Check sheet for the drawn part. Datum: minimum x, y, z corner. Units: mm. A direction names the side the tool comes from. Coordinates: 2 decimals unless noted, no trailing zeros. Write each loop counter-clockwise with the first axis right and the second up, starting at its lowest first coordinate (ties: lowest second). Pieces come first, ordered by that corner, then holes. Notation, with made-up numbers: (-34.5, 67.5) - (14.5, 67.5) arc R14 cw to (14.5, 76.5) - close; hole circle Ø9 at (-28, -29). An arc over 180 degrees is marked (long way). Answer as CSV lines item,"result". Start each with the question number.
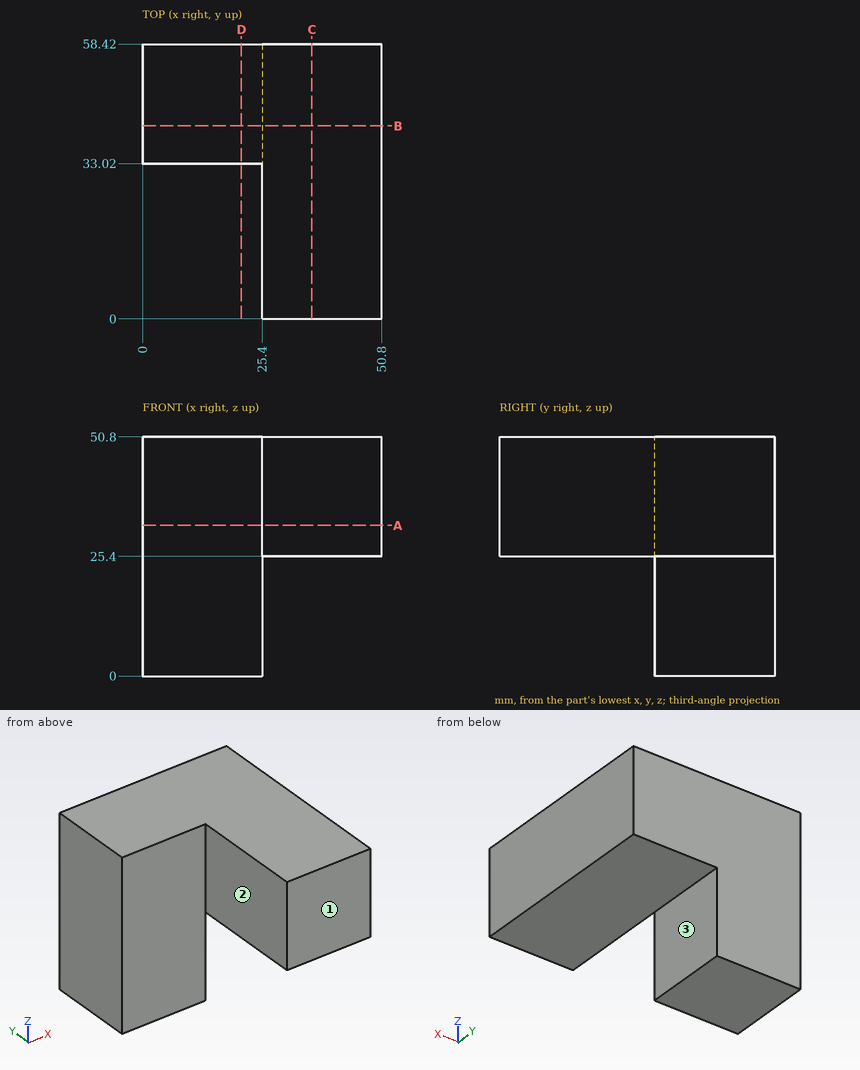
(1) Material ranges on probe 1 along X at (y, z) = (11.5, 26); probe 2 along X at (y, z) = (49.5, 4), recorded low to high. Write a range as from..to.
(2) Go/stop test with flat-tipped pins: P1, Ø12.5, axis at x = 10, z = 13, coming from the -Y side; P2, Ø3, axis at x = 29.5, z = 24.5, coming from the -Y side; P3, Ø2, axis at x = 36, y = 31.5, coming from the -Z side; P4, Ø7.5, axis at y = 12.5, z = 39.5, coming from the -X side. Record where each tip stops, or that it passes through.
(3) Cross-section at D-D on x = 21. Record the boundary of the cut face in (y, z).
(4) Cross-section at B-B on y = 41. Record the boundary of the cut face in (x, z), plus the area to 3 significant figures.
(5) Tool access check on the marked faces 1, 2 and 3. Record the directions out of +Z, -Z, +X, -X, +Y, -Y that give a thin tool (end or side, any length) a straight path to the whole face; none if there is none.
(6) Cross-section at C-C on x = 36. Record the boundary of the cut face in (y, z).
(7) Cross-section at A-A on z = 32. Record the boundary of the cut face in (x, y), plus the area to 3 significant figures.
Checked values:
1,probe 1,"25.4..50.8"
1,probe 2,"0..25.4"
2,P1,"y = 33.02"
2,P2,"y = 0"
2,P3,"z = 25.4"
2,P4,"x = 25.4"
3,outline,"(33.02, 0) - (58.42, 0) - (58.42, 50.8) - (33.02, 50.8) - close"
4,outline,"(0, 0) - (25.4, 0) - (25.4, 25.4) - (50.8, 25.4) - (50.8, 50.8) - (0, 50.8) - close"
4,area,"1,940 mm^2"
5,face 1,"+Z, -Z, +X, -X, -Y"
5,face 2,"+Z, -Z, -X, -Y"
5,face 3,"-Z, +X, +Y, -Y"
6,outline,"(0, 25.4) - (58.42, 25.4) - (58.42, 50.8) - (0, 50.8) - close"
7,outline,"(0, 33.02) - (25.4, 33.02) - (25.4, 0) - (50.8, 0) - (50.8, 58.42) - (0, 58.42) - close"
7,area,"2,130 mm^2"
